For this review, take the finished solid that the model builds, in its own axes (mm). Coordinates: 2 decimals unless noted, no trailing zeros. Write each loop counter-clockwise with the first axis right and the second up, starting at its lowest first coordinate (ties: lowest second). Pieces come first, ordered by that corner, then holes. Notation, with made-up numbers: M 16,-17 L 70,-17 A28 ccw 70,16 Z; hole C -30,87 d5. An arc over 180 degrees is marked long. Return JSON: item names as keys, results as strings.
```python
from build123d import *

# Parameters (mm, degrees)
SHAFT_BOSS_DEPTH = 914.4
FILLET1_R        = 0.508


with BuildPart() as part:
    # Sketch1 → Shaft Boss (new body)
    with BuildSketch(Plane.XY):
        Polygon((0, 5.499261314), (-4.7625, 2.749630657), (-4.7625, -2.749630657), (0, -5.499261314), (4.7625, -2.749630657), (4.7625, 2.749630657), align=None)
    extrude(amount=SHAFT_BOSS_DEPTH)

    # Fillet1
    fillet1_edges = [part.edges().sort_by_distance(p)[0] for p in [
        (4.7625, 2.749630657, 457.2),
        (4.7625, -2.749630657, 457.2),
        (0, -5.499261314, 457.2),
        (-4.7625, -2.749630657, 457.2),
        (-4.7625, 2.749630657, 457.2),
        (0, 5.499261314, 457.2),
    ]]
    fillet(fillet1_edges, radius=FILLET1_R)


solid = part.part
```
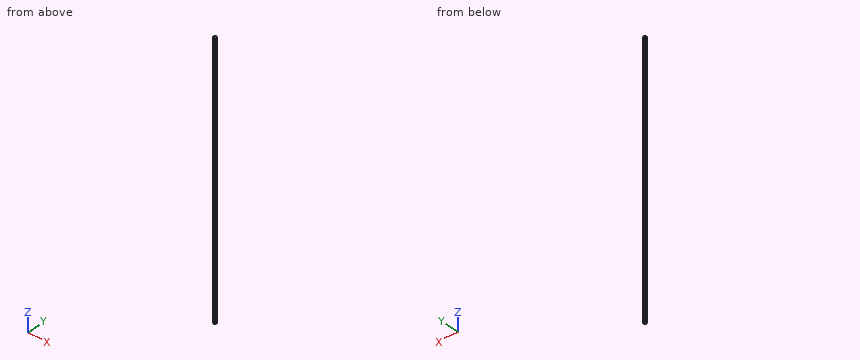
1. Wall thickness on L1, parallel to Y at x = -1, z = 472.5; L2, parallel to Y at x = -1.75, z = 66.5; L3, parallel to X at y = -2.75, z = 451: over which ranges is each line inside the solid? List them lowest first. Write a range as from..to.
Checks:
{"L1": "-4.92..4.92", "L2": "-4.49..4.49", "L3": "-4.67..4.67"}
2. Clearance check with a flat-ended pin moving along its axis: pin 1 Ø1.5 at (y, z) = (-4, 526) entering from +X. State where the tip first meets the part, or that it passes through.
Checks:
{"pin 1": "x = 3.9"}
3. We need section B-B (x = 2.25). State the section outline as (y, z) points, plus the area to 3 significant figures.
Checks:
{"outline": "M -4.2,0 L 4.2,0 L 4.2,914.4 L -4.2,914.4 Z", "area": "7,680 mm2"}
4. We need section A-A (z = 287). State the section outline as (x, y) points.
Checks:
{"outline": "M -4.76,-2.46 A0.51 ccw -4.51,-2.9 L -0.25,-5.35 A0.51 ccw 0.25,-5.35 L 4.51,-2.9 A0.51 ccw 4.76,-2.46 L 4.76,2.46 A0.51 ccw 4.51,2.9 L 0.25,5.35 A0.51 ccw -0.25,5.35 L -4.51,2.9 A0.51 ccw -4.76,2.46 Z"}
